Model file for the job. Use its own axes, mm. Face numbers are marked on the shaded views. A direction names the side the tool comes from. Round coordinates to 2 decimals unless told otherwise and drop trailing zeros. Loops run counter-clockwise (first coordinate to the right, second up) from the corner with the lowest first, then second, coordinate; pieces in that order, holes last. Notation, with made-up numbers: (14, 38) -> (56, 38) arc R35 ccw to (56, 72) -> close; hole circle Ø4 at (-35.75, 44). An arc over 180 degrees is marked (long way). Use a Markdown table: item, result.
from build123d import *

# Parameters (mm, degrees)
F1_DEPTH      = 75
F1_DEPTH_BACK = 75
F3_START      = 30
F2_W          = 100
F2_H          = 200
F3_DEPTH      = 170


with BuildPart() as f1:
    # F0 (on Front) → F1 (new body, two sides)
    with BuildSketch(Plane.XZ) as f1_sk:
        with BuildLine():
            Line((110, 0), (0, 0))
            Line((0, 0), (0, -160))
            Line((0, -160), (30, -160))
            Line((30, -160), (30, -140))
            Line((30, -140), (50, -140))
            Line((50, -140), (50, -120))
            Line((50, -120), (70, -120))
            Line((70, -120), (70, -100))
            Line((70, -100), (90, -100))
            Line((90, -100), (90, -80))
            Line((90, -80), (110, -80))
            Line((110, -80), (110, -58.5))
            ThreePointArc((110, -58.5), (91.5, -40), (110, -21.5))
            Line((110, -21.5), (110, 0))
        make_face()
    extrude(amount=F1_DEPTH)
    extrude(f1_sk.sketch, amount=-F1_DEPTH_BACK)

    # F2 (on Right) → F3 (cut)
    with BuildSketch(Plane.YZ.offset(F3_START)):
        with Locations((0, -90)):
            Rectangle(F2_W, F2_H)
    extrude(amount=F3_DEPTH, mode=Mode.SUBTRACT)


solid = f1.part
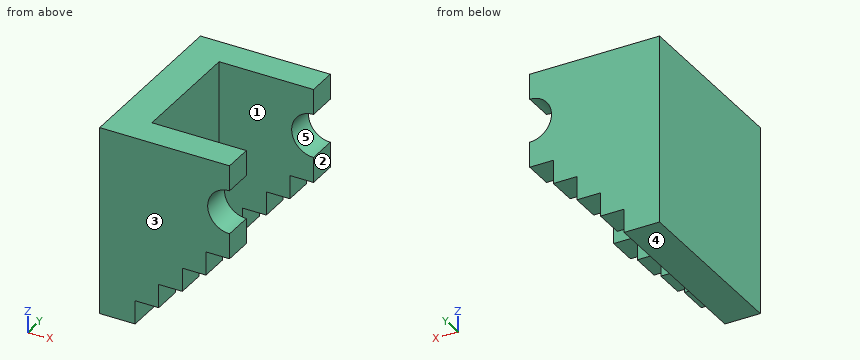
Q1. Band-saw the part on C-C, the plane y = 56. Give the cut face in (x, z), plus the area to 3 significant figures.
Results list:
| item | result |
|---|---|
| outline | (0, -160) -> (30, -160) -> (30, -140) -> (50, -140) -> (50, -120) -> (70, -120) -> (70, -100) -> (90, -100) -> (90, -80) -> (110, -80) -> (110, -58.5) arc R18.5 cw to (110, -21.5) -> (110, 0) -> (0, 0) -> close |
| area | 13,100 mm² |
Q2. Drill centre lines: L1, parallel to Y at x = 47, z = -50; L2, parallel to X at y = -18, z = -80; L3, parallel to X at y = 67.5, z = -130. Where is each one in solid material? Low to high. Write a range as from..to.
Results list:
| item | result |
|---|---|
| L1 | y = -75..-50, 50..75 |
| L2 | x = 0..30 |
| L3 | x = 0..50 |
Q3. Flat gauge pins, fed straight in: pin 1 (6 mm diameter, centred on y = 61.5, z = -93, fed in from +X); pin 2 (22 mm diameter, centred on x = 98, y = 65.5, fed in from -Z); pin 3 (16 mm diameter, centred on y = -62.5, z = -113, fed in from +X). Where does each tip first touch, or does it go through?
Results list:
| item | result |
|---|---|
| pin 1 | stops at x = 90 |
| pin 2 | stops at z = -100 |
| pin 3 | stops at x = 70 |
Q4. Band-saw the part on A-A, the plane x = 48. Give the cut face in (y, z).
Results list:
| item | result |
|---|---|
| outline | (-75, -140) -> (-50, -140) -> (-50, 0) -> (-75, 0) -> close; (50, -140) -> (75, -140) -> (75, 0) -> (50, 0) -> close |
Q5. Band-saw the part on B-B, the plane z = -131. Give the cut face in (x, y), plus the area to 3 significant figures.
Results list:
| item | result |
|---|---|
| outline | (0, -75) -> (50, -75) -> (50, -50) -> (30, -50) -> (30, 50) -> (50, 50) -> (50, 75) -> (0, 75) -> close |
| area | 5,500 mm² |
Q6. Pull direction Z, two halves, no side cores. Call the marked faces 3, 4 and 5: released by +Z, released by -Z, zero draft, split by the parting line, or undercut.
Results list:
| item | result |
|---|---|
| face 3 | zero draft |
| face 4 | released by -Z |
| face 5 | undercut |
Q7. Band-saw the part on D-D, the plane z = -97. Give the cut face in (x, y), plus the area to 3 significant figures.
Results list:
| item | result |
|---|---|
| outline | (0, -75) -> (90, -75) -> (90, -50) -> (30, -50) -> (30, 50) -> (90, 50) -> (90, 75) -> (0, 75) -> close |
| area | 7,500 mm² |
Q8. Tool access for the marked faces 1 and 2: list every direction of +Z, -Z, +X, -X, +Y, -Y with a clear straight run to the whole face (end or side of a thin tool).
Results list:
| item | result |
|---|---|
| face 1 | +Z, -Z, +X |
| face 2 | +Z, -Z, +X, +Y, -Y |
